from build123d import *

# Parameters (mm, degrees)
F0_W         = 50
F0_H         = 10
F0_R         = 1.6
F1_DEPTH     = 5
F2_W         = 15
F2_H         = 10
F2_R         = 1.6
F3_DEPTH     = 10
F5_R         = 5
F6_R         = 4.99999
F4_R         = 6
F7_DEPTH     = 25
F8_T1_DEPTH  = 12.50001
F8_T3_DEPTH  = 5
F8_T5_DEPTH  = 5
F8_T7_DEPTH  = 12.50001
F8_T9_DEPTH  = 2.50001
F8_T12_ANGLE = 90
F8_T14_ANGLE = 90
F8_T16_ANGLE = 90
F8_T18_ANGLE = 90
F8_T20_ANGLE = 90
F8_T22_ANGLE = 90
F8_T24_ANGLE = 90
F8_T26_ANGLE = 90
F8_T31_DEPTH = 7.5
F8_T35_DEPTH = 15.00001
F8_T42_DEPTH = 15.00001
F8_T46_DEPTH = 7.5
F8_T53_DEPTH = 15.00001
F8_T57_DEPTH = 7.5
F8_T64_DEPTH = 7.5
F8_T68_DEPTH = 15.00001
F9_W         = 10
F9_H         = 2
F10_DEPTH    = 10
F11_R        = 4.99999


# Not quite as in the source:
# - a fillet or chamfer that OpenCascade refuses, or shapes differently, is made with other operations: its cross-section is extruded or revolved along the edge and cut away or added
# - a fillet or chamfer is up to 0.001 mm smaller than in the source, because OpenCascade refuses the exact size


with BuildPart() as f1:
    # F0 (on Top) → F1 (new body)
    with BuildSketch(Plane.XY):
        Rectangle(F0_W, F0_H)
        with Locations((-16, 0)):
            Circle(F0_R, mode=Mode.SUBTRACT)
        with Locations((16, 0)):
            Circle(F0_R, mode=Mode.SUBTRACT)
    extrude(amount=F1_DEPTH)

    # F2 (on face) → F3 (join)
    with BuildSketch(Plane.XY.offset(5)):
        Rectangle(F2_W, F2_H)
        with Locations((-3.9, 0)):
            Circle(F2_R, mode=Mode.SUBTRACT)
        with Locations((3.9, 0)):
            Circle(F2_R, mode=Mode.SUBTRACT)
        with Locations((3.9, 0)):
            Circle(F2_R)
        with Locations((-3.9, 0)):
            Circle(F2_R)
    extrude(amount=F3_DEPTH)

    # F5
    f5_edges = [f1.edges().sort_by_distance(p)[0] for p in [
        (7.5, 0, 15),
        (-7.5, 0, 15),
    ]]
    fillet(f5_edges, radius=F5_R)

    # F6 (radius 5 in the source; OpenCascade refuses exactly that, so slightly less here)
    f6_edges = [f1.edges().sort_by_distance(p)[0] for p in [
        (-25, 0, 5),
        (25, 0, 5),
    ]]
    fillet(f6_edges, radius=F6_R)

    # F4 (on face) → F7 (cut)
    with BuildSketch(Plane(origin=(0, 5, 0), x_dir=(-1, 0, 0), z_dir=(0, 1, 0))):
        with Locations((0, 7.5)):
            Circle(F4_R)
    extrude(amount=-F7_DEPTH, mode=Mode.SUBTRACT)

    # F8: fillet of radius 1 on 18 edges, made by hand

    # F8_s2 → F8_t1 (cut)
    with BuildSketch(Plane.YZ.offset(7.5)):
        with BuildLine():
            ThreePointArc((-5, 4), (-4.7071067812, 4.7071067812), (-4, 5))
            Line((-4, 5), (-5, 5))
            Line((-5, 5), (-5, 4))
        make_face()
        with BuildLine():
            ThreePointArc((4, 5), (4.7071067812, 4.7071067812), (5, 4))
            Line((5, 4), (5, 5))
            Line((5, 5), (4, 5))
        make_face()
    extrude(amount=F8_T1_DEPTH, mode=Mode.SUBTRACT)

    # F8_s4 → F8_t3 (cut)
    with BuildSketch(Plane.XY.offset(5)):
        with BuildLine():
            ThreePointArc((6.5, -5), (7.2071067812, -4.7071067812), (7.5, -4))
            Line((7.5, -4), (7.5, -5))
            Line((7.5, -5), (6.5, -5))
        make_face()
        with BuildLine():
            ThreePointArc((-6.5, -5), (-7.2071067812, -4.7071067812), (-7.5, -4))
            Line((-7.5, -4), (-7.5, -5))
            Line((-7.5, -5), (-6.5, -5))
        make_face()
        with BuildLine():
            ThreePointArc((7.5, 4), (7.2071067812, 4.7071067812), (6.5, 5))
            Line((6.5, 5), (7.5, 5))
            Line((7.5, 5), (7.5, 4))
        make_face()
        with BuildLine():
            ThreePointArc((-7.5, 4), (-7.2071067812, 4.7071067812), (-6.5, 5))
            Line((-6.5, 5), (-7.5, 5))
            Line((-7.5, 5), (-7.5, 4))
        make_face()
    extrude(amount=F8_T3_DEPTH, mode=Mode.SUBTRACT)

    # F8_s6 → F8_t5 (cut)
    with BuildSketch(Plane.YZ.offset(-2.5)):
        with BuildLine():
            ThreePointArc((-5, 14), (-4.7071067812, 14.7071067812), (-4, 15))
            Line((-4, 15), (-5, 15))
            Line((-5, 15), (-5, 14))
        make_face()
        with BuildLine():
            ThreePointArc((4, 15), (4.7071067812, 14.7071067812), (5, 14))
            Line((5, 14), (5, 15))
            Line((5, 15), (4, 15))
        make_face()
    extrude(amount=F8_T5_DEPTH, mode=Mode.SUBTRACT)

    # F8_s8 → F8_t7 (cut)
    with BuildSketch(Plane.YZ.offset(-20.00001)):
        with BuildLine():
            ThreePointArc((-5, 4), (-4.7071067812, 4.7071067812), (-4, 5))
            Line((-4, 5), (-5, 5))
            Line((-5, 5), (-5, 4))
        make_face()
        with BuildLine():
            ThreePointArc((4, 5), (4.7071067812, 4.7071067812), (5, 4))
            Line((5, 4), (5, 5))
            Line((5, 5), (4, 5))
        make_face()
    extrude(amount=F8_T7_DEPTH, mode=Mode.SUBTRACT)

    # F8_s10 → F8_t9 (cut)
    with BuildSketch(Plane.XY.offset(-2.5)):
        with BuildLine():
            ThreePointArc((-25, 4), (-24.7071067812, 4.7071067812), (-24, 5))
            Line((-24, 5), (-25, 5))
            Line((-25, 5), (-25, 4))
        make_face()
        with BuildLine():
            ThreePointArc((25, 4), (24.7071067812, 4.7071067812), (24, 5))
            Line((24, 5), (25, 5))
            Line((25, 5), (25, 4))
        make_face()
        with BuildLine():
            ThreePointArc((-24, -5), (-24.7071067812, -4.7071067812), (-25, -4))
            Line((-25, -4), (-25, -5))
            Line((-25, -5), (-24, -5))
        make_face()
        with BuildLine():
            ThreePointArc((24, -5), (24.7071067812, -4.7071067812), (25, -4))
            Line((25, -4), (25, -5))
            Line((25, -5), (24, -5))
        make_face()
    extrude(amount=F8_T9_DEPTH, mode=Mode.SUBTRACT)

    # F8_s11 → F8_t12 (revolve, cut)
    with BuildSketch(Plane.XY.offset(1e-05)):
        with BuildLine():
            ThreePointArc((24, -5), (24.7071067812, -4.7071067812), (25, -4))
            Line((25, -4), (25, -5))
            Line((25, -5), (24, -5))
        make_face()
    revolve(axis=Axis((20.00001, -5, 1e-05), (0, -1, 0)), revolution_arc=F8_T12_ANGLE, mode=Mode.SUBTRACT)

    # F8_s13 → F8_t14 (revolve, cut)
    with BuildSketch(Plane.XY.offset(10)):
        with BuildLine():
            ThreePointArc((6.5, -5), (7.2071067812, -4.7071067812), (7.5, -4))
            Line((7.5, -4), (7.5, -5))
            Line((7.5, -5), (6.5, -5))
        make_face()
    revolve(axis=Axis((2.5, -5, 10), (0, -1, 0)), revolution_arc=F8_T14_ANGLE, mode=Mode.SUBTRACT)

    # F8_s15 → F8_t16 (revolve, cut)
    with BuildSketch(Plane.XY.offset(10)):
        with BuildLine():
            ThreePointArc((-6.5, -5), (-7.2071067812, -4.7071067812), (-7.5, -4))
            Line((-7.5, -4), (-7.5, -5))
            Line((-7.5, -5), (-6.5, -5))
        make_face()
    revolve(axis=Axis((-2.5, -5, 10), (0, 1, 0)), revolution_arc=F8_T16_ANGLE, mode=Mode.SUBTRACT)

    # F8_s17 → F8_t18 (revolve, cut)
    with BuildSketch(Plane.YZ.offset(-20.00001)):
        with BuildLine():
            ThreePointArc((-5, 4), (-4.7071067812, 4.7071067812), (-4, 5))
            Line((-4, 5), (-5, 5))
            Line((-5, 5), (-5, 4))
        make_face()
    revolve(axis=Axis((-20.00001, -5, 1e-05), (0, -1, 0)), revolution_arc=F8_T18_ANGLE, mode=Mode.SUBTRACT)

    # F8_s19 → F8_t20 (revolve, cut)
    with BuildSketch(Plane.XY.offset(10)):
        with BuildLine():
            ThreePointArc((7.5, 4), (7.2071067812, 4.7071067812), (6.5, 5))
            Line((6.5, 5), (7.5, 5))
            Line((7.5, 5), (7.5, 4))
        make_face()
    revolve(axis=Axis((2.5, 5, 10), (0, -1, 0)), revolution_arc=F8_T20_ANGLE, mode=Mode.SUBTRACT)

    # F8_s21 → F8_t22 (revolve, cut)
    with BuildSketch(Plane.XY.offset(1e-05)):
        with BuildLine():
            ThreePointArc((25, 4), (24.7071067812, 4.7071067812), (24, 5))
            Line((24, 5), (25, 5))
            Line((25, 5), (25, 4))
        make_face()
    revolve(axis=Axis((20.00001, 5, 1e-05), (0, -1, 0)), revolution_arc=F8_T22_ANGLE, mode=Mode.SUBTRACT)

    # F8_s23 → F8_t24 (revolve, cut)
    with BuildSketch(Plane.XY.offset(10)):
        with BuildLine():
            ThreePointArc((-7.5, 4), (-7.2071067812, 4.7071067812), (-6.5, 5))
            Line((-6.5, 5), (-7.5, 5))
            Line((-7.5, 5), (-7.5, 4))
        make_face()
    revolve(axis=Axis((-2.5, 5, 10), (0, 1, 0)), revolution_arc=F8_T24_ANGLE, mode=Mode.SUBTRACT)

    # F8_s25 → F8_t26 (revolve, cut)
    with BuildSketch(Plane.YZ.offset(-20.00001)):
        with BuildLine():
            ThreePointArc((4, 5), (4.7071067812, 4.7071067812), (5, 4))
            Line((5, 4), (5, 5))
            Line((5, 5), (4, 5))
        make_face()
    revolve(axis=Axis((-20.00001, 5, 1e-05), (0, -1, 0)), revolution_arc=F8_T26_ANGLE, mode=Mode.SUBTRACT)


with BuildPart() as f8_tool29:
    # F8_s30 → F8_t31 (new body)
    with BuildSketch(Plane.XY.offset(2.5)):
        with BuildLine():
            ThreePointArc((6.5, -5), (7.2071067812, -4.7071067812), (7.5, -4))
            Line((7.5, -4), (7.5, -5))
            Line((7.5, -5), (6.5, -5))
        make_face()
    extrude(amount=F8_T31_DEPTH)

    split(bisect_by=Plane.XY.offset(5), keep=Keep.BOTTOM)


with BuildPart() as f8_tool33:
    # F8_s34 → F8_t35 (new body)
    with BuildSketch(Plane.YZ.offset(5)):
        with BuildLine():
            ThreePointArc((-5, 4), (-4.7071067812, 4.7071067812), (-4, 5))
            Line((-4, 5), (-5, 5))
            Line((-5, 5), (-5, 4))
        make_face()
    extrude(amount=F8_T35_DEPTH)

    split(bisect_by=Plane.YZ.offset(7.5), keep=Keep.BOTTOM)


with BuildPart() as f8_tool29_1:
    add(f8_tool29.part)

    # F8_t37: intersect F8_tool33
    add(f8_tool33.part, mode=Mode.INTERSECT)


with BuildPart() as f1_1:
    add(f1.part)

    # F8_t27: cut F8_tool29
    add(f8_tool29_1.part, mode=Mode.SUBTRACT)


with BuildPart() as f8_tool40:
    # F8_s41 → F8_t42 (new body)
    with BuildSketch(Plane.YZ.offset(-20.00001)):
        with BuildLine():
            ThreePointArc((-5, 4), (-4.7071067812, 4.7071067812), (-4, 5))
            Line((-4, 5), (-5, 5))
            Line((-5, 5), (-5, 4))
        make_face()
    extrude(amount=F8_T42_DEPTH)

    split(bisect_by=Plane.YZ.offset(-7.5), keep=Keep.TOP)


with BuildPart() as f8_tool44:
    # F8_s45 → F8_t46 (new body)
    with BuildSketch(Plane.XY.offset(2.5)):
        with BuildLine():
            ThreePointArc((-6.5, -5), (-7.2071067812, -4.7071067812), (-7.5, -4))
            Line((-7.5, -4), (-7.5, -5))
            Line((-7.5, -5), (-6.5, -5))
        make_face()
    extrude(amount=F8_T46_DEPTH)

    split(bisect_by=Plane.XY.offset(5), keep=Keep.BOTTOM)


with BuildPart() as f8_tool40_1:
    add(f8_tool40.part)

    # F8_t48: intersect F8_tool44
    add(f8_tool44.part, mode=Mode.INTERSECT)


with BuildPart() as f1_2:
    add(f1_1.part)

    # F8_t38: cut F8_tool40
    add(f8_tool40_1.part, mode=Mode.SUBTRACT)


with BuildPart() as f8_tool51:
    # F8_s52 → F8_t53 (new body)
    with BuildSketch(Plane.YZ.offset(-5)):
        with BuildLine():
            ThreePointArc((4, 5), (4.7071067812, 4.7071067812), (5, 4))
            Line((5, 4), (5, 5))
            Line((5, 5), (4, 5))
        make_face()
    extrude(amount=-F8_T53_DEPTH)

    split(bisect_by=Plane.YZ.offset(-7.5), keep=Keep.TOP)


with BuildPart() as f8_tool55:
    # F8_s56 → F8_t57 (new body)
    with BuildSketch(Plane.XY.offset(2.5)):
        with BuildLine():
            ThreePointArc((-7.5, 4), (-7.2071067812, 4.7071067812), (-6.5, 5))
            Line((-6.5, 5), (-7.5, 5))
            Line((-7.5, 5), (-7.5, 4))
        make_face()
    extrude(amount=F8_T57_DEPTH)

    split(bisect_by=Plane.XY.offset(5), keep=Keep.BOTTOM)


with BuildPart() as f8_tool51_1:
    add(f8_tool51.part)

    # F8_t59: intersect F8_tool55
    add(f8_tool55.part, mode=Mode.INTERSECT)


with BuildPart() as f1_3:
    add(f1_2.part)

    # F8_t49: cut F8_tool51
    add(f8_tool51_1.part, mode=Mode.SUBTRACT)


with BuildPart() as f8_tool62:
    # F8_s63 → F8_t64 (new body)
    with BuildSketch(Plane.XY.offset(2.5)):
        with BuildLine():
            ThreePointArc((7.5, 4), (7.2071067812, 4.7071067812), (6.5, 5))
            Line((6.5, 5), (7.5, 5))
            Line((7.5, 5), (7.5, 4))
        make_face()
    extrude(amount=F8_T64_DEPTH)

    split(bisect_by=Plane.XY.offset(5), keep=Keep.BOTTOM)


with BuildPart() as f8_tool66:
    # F8_s67 → F8_t68 (new body)
    with BuildSketch(Plane.YZ.offset(20.00001)):
        with BuildLine():
            ThreePointArc((4, 5), (4.7071067812, 4.7071067812), (5, 4))
            Line((5, 4), (5, 5))
            Line((5, 5), (4, 5))
        make_face()
    extrude(amount=-F8_T68_DEPTH)

    split(bisect_by=Plane.YZ.offset(7.5), keep=Keep.BOTTOM)


with BuildPart() as f8_tool62_1:
    add(f8_tool62.part)

    # F8_t70: intersect F8_tool66
    add(f8_tool66.part, mode=Mode.INTERSECT)


with BuildPart() as f1_4:
    add(f1_3.part)

    # F8_t60: cut F8_tool62
    add(f8_tool62_1.part, mode=Mode.SUBTRACT)

    # F9 (on face) → F10 (join)
    with BuildSketch(Plane(origin=(0, 0, 0), x_dir=(1, 0, 0), z_dir=(0, 0, -1))):
        with Locations((-16, -4)):
            Rectangle(F9_W, F9_H)
        with Locations((16, -4)):
            Rectangle(F9_W, F9_H)
    extrude(amount=F10_DEPTH)

    # F11 (radius 5 in the source; OpenCascade refuses exactly that, so slightly less here)
    f11_edges = [f1_4.edges().sort_by_distance(p)[0] for p in [
        (11, 4, -10),
        (21, 4, -10),
        (-21, 4, -10),
        (-11, 4, -10),
    ]]
    fillet(f11_edges, radius=F11_R)


solid = f1_4.part
Verification items for the finished model (mm, model axes). A direction names the side the tool comes from. Coordinates: 2 decimals unless noted, no trailing zeros. Loops run counter-clockwise (first coordinate to the right, second up) from the corner with the lowest first, then second, coordinate; pieces in that order, holes last. Notation, with made-up numbers: (88, 40.5) -> (137, 40.5) arc R13 cw to (137, 54.5) -> close; hole circle Ø11 at (-25.75, 55.25). An arc over 180 degrees is marked (long way). Write each question's results on one line, items separated by ' | '.
Item 1: Material ranges on L1, parallel to X at y = 4.25, z = -4; L2, parallel to Y at x = -16, z = 1.9; L3, parallel to X at y = 0, z = 9, recorded low to high.
Found:
L1: x = -21 to -11, 11 to 21 | L2: y = -5 to -1.6, 1.6 to 5 | L3: x = -7.5 to -5.81, 5.81 to 7.5
Item 2: Section check A-A, the plane y = 0. Count the separate pieces of the cut face and the enclosed holes in it, plus the area to 3 significant figures.
Found:
separate pieces: 3 | enclosed holes: 1 | area: 233 mm2
Item 3: Tool access check on faces 4 (the face through (7.215, 4.699, 6.958)), 5 (the face through (-7.5, 0, 7)), 6 (the face through (-13.345, -4.715, 4.699)). Record the directions out of +Z, -Z, +X, -X, +Y, -Y that give a thin tool (end or side, any length) a straight path to the whole face; none if there is none.
Found:
face 4: +Z, +X, +Y | face 5: +Z, -X, +Y, -Y | face 6: +Z, -X, -Y
Item 4: Mould release check, pull along Z, two halves, no side actions. Record for faces 1 (the face through (5.994, 0.07, 7.764)), 2 (the face through (-12, 4, -8)), 3 (the face through (24, 0, 3)): +Z half, -Z half, draft (parallel to the pull), parting line (faces both ways), or undercut.
Found:
face 1: undercut | face 2: -Z half | face 3: +Z half
Item 5: Section check C-C, the plane x = 0. Enter the section's corners in (y, z), plus the area to 3 significant figures.
Found:
outline: (-5, 0) -> (5, 0) -> (5, 1.5) -> (-5, 1.5) -> close; (-5, 13.5) -> (5, 13.5) -> (5, 14) arc R1 ccw to (4, 15) -> (-4, 15) arc R1 ccw to (-5, 14) -> close | area: 29.6 mm2
Item 6: Section check B-B, the plane z = 7.5. Enter the section's corners in (x, y), plus the area to 3 significant figures.
Found:
outline: (-7.5, -4) arc R1 ccw to (-6.5, -5) -> (-6, -5) -> (-6, 5) -> (-6.5, 5) arc R1 ccw to (-7.5, 4) -> close; (6, -5) -> (6.5, -5) arc R1 ccw to (7.5, -4) -> (7.5, 4) arc R1 ccw to (6.5, 5) -> (6, 5) -> close | area: 29.1 mm2
Item 7: Gauge pin test, flat ends, axial feed: pin 1 (8 mm diameter, centred on x = -16.5, z = -6, fed in from -Y); pin 2 (2 mm diameter, centred on x = 13.5, y = 0, fed in from +Z); pin 3 (1 mm diameter, centred on y = 3.5, z = -2.5, fed in from +X); pin 4 (6 mm diameter, centred on x = -8.5, z = 7, fed in from -Y). Record the tip position at first contact, or that the pin passes through.
Found:
pin 1: stops at y = 3 | pin 2: stops at z = 5 | pin 3: stops at x = 21 | pin 4: stops at y = -5
